The model under review builds one solid part; all positions refer to its coordinate system, in mm. Coordinates: 2 decimals unless noted, no trailing zeros. Write each loop counter-clockwise with the first axis right and the second up, starting at its lowest first coordinate (ties: lowest second). Pieces come first, ordered by that corner, then holes. Notation, with made-up numbers: (70.5, -26.5) - (129.5, -26.5) arc R21 cw to (129.5, -18.5) - close; hole circle Ø9 at (51, 80). An arc over 180 degrees is marked (long way). Put each result on its own line as item: value.
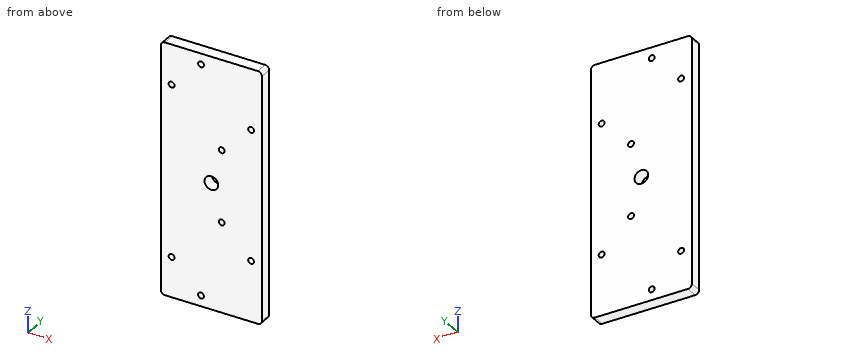
Autodesk Inventor part; units mm, degrees
ref_plane "YZ Plane" through (0, 0, 0) normal (1, 0, 0) x (0, 1, 0)
ref_plane "XZ Plane" through (0, 0, 0) normal (0, 1, 0) x (-1, 0, 0)
ref_plane "XY Plane" through (0, 0, 0) normal (0, 0, 1) x (1, 0, 0)
sketch "Sketch1" plane through (0, 0, 0) normal (0, 1, 0) x (-1, 0, 0)
  line L0 (-25, 62.5) -> (25, 62.5)
  line L1 (25, 62.5) -> (25, -62.5)
  line L2 (25, -62.5) -> (-25, -62.5)
  line L3 (-25, -62.5) -> (-25, 62.5)
  line L4 (-25, 62.5) -> (25, -62.5) construction
  line L5 (25, 62.5) -> (-25, -62.5) construction
  point P0 (0, 0)
  dimension "d0" = 125
  dimension "d1" = 50
extrude "Extrusion1" add sketch "Sketch1" along normal blind 6
sketch "Sketch3" plane through (0, 6, 0) normal (0, 1, 0) x (1, 0, 0)
  line L0 (25, 62.5) -> (-25, 62.5)
  line L1 (-25, -62.5) -> (25, -62.5)
  line L2 (-19.6668, -42.6187) -> (-5.1187, -57.1668)
  line L3 (-5.1187, -57.1668) -> (19.6668, -32.3813)
  line L4 (19.6668, -32.3813) -> (5.1187, -17.8332)
  line L5 (5.1187, -17.8332) -> (-19.6668, -42.6187)
  line L6 (25, -62.5) -> (25, 62.5)
  line L7 (-25, 62.5) -> (-25, -62.5)
  line L8 (5.1187, 17.8332) -> (19.6668, 32.3813)
  line L9 (19.6668, 32.3813) -> (-5.1187, 57.1668)
  line L10 (-5.1187, 57.1668) -> (-19.6668, 42.6187)
  line L11 (-19.6668, 42.6187) -> (5.1187, 17.8332)
  circle A0 centre (-19.6668, -42.6187) radius 1.45
  circle A1 centre (5.1187, -17.8332) radius 1.45
  circle A2 centre (19.6668, -32.3813) radius 1.45
  circle A3 centre (-5.1187, -57.1668) radius 1.45
  circle A4 centre (-19.6668, 42.6187) radius 1.45
  circle A5 centre (-5.1187, 57.1668) radius 1.45
  circle A6 centre (19.6668, 32.3813) radius 1.45
  circle A7 centre (5.1187, 17.8332) radius 1.45
  point P0 (0, 0)
  point P1 (0, -37.5)
  point P2 (0, 37.5)
  point P3 (0, -62.5)
  point P4 (0, 62.5)
  dimension "d5" = 125
  dimension "d7" = 35.052
  dimension "d8" = 20.574
  dimension "d9" = 50
  dimension "d10" = 10.287
  dimension "d11" = 17.526
  dimension "d12" = 35.052
  dimension "d13" = 20.574
  dimension "d14" = 17.526
  dimension "d15" = 10.287
  dimension "d16" = 2.9
  dimension "d17" = 2.9
  dimension "d18" = 2.9
  dimension "d19" = 2.9
  dimension "d20" = 2.9
  dimension "d21" = 2.9
  dimension "d22" = 2.9
  dimension "d23" = 2.9
  dimension "d24" = 25
  dimension "d25" = 25
extrude "Extrusion2" cut sketch "Sketch3" against normal through all contours L5 A0 L2 | L2 A0 L5 | A3 L3 L2 | L2 L3 A3 | A1 L4 L5 | L5 L4 A1 | A2 L4 L3 | L3 L4 A2 | L11 A7 L8 | L8 A7 L11 | A6 L9 L8 | L8 L9 A6 | A4 L10 L11 | L11 L10 A4 | A5 L10 L9 | L9 L10 A5
hole "Hole1" at (0, 6, 0) direction (0, -1, 0) diameter 6.756 end through all
fillet "Fillet1" radius 2 4 edges at (25, 3, 62.5) (25, 3, -62.5) (-25, 3, -62.5) (-25, 3, 62.5)
properties part number "ShuttleValveShelf"
1. To check wall thickness, follow probe 1 along Z at (x, y) = (19.5, 3.8); probe 2 along X at (y, z) = (5.75, 18); probe 3 along Z at (x, y) = (20.5, 3.7). State the ranges of each line that lie inside material, in increasing order.
Determined:
probe 1: z = -62.5 to -33.82, -30.94 to 30.94, 33.82 to 62.5
probe 2: x = -25 to 3.68, 6.56 to 25
probe 3: z = -62.5 to -33.57, -31.19 to 31.19, 33.57 to 62.5
2. Consider section A-A on z = 0. State the section outline as (x, y) points, plus the area to 3 significant figures.
Determined:
outline: (-25, 0) - (-3.38, 0) - (-3.38, 6) - (-25, 6) - close; (3.38, 0) - (25, 0) - (25, 6) - (3.38, 6) - close
area: 259 mm^2
3. Consider section B-B on x = 0. State the section outline as (y, z) points.
Determined:
outline: (0, -62.5) - (6, -62.5) - (6, -3.38) - (0, -3.38) - close; (0, 3.38) - (6, 3.38) - (6, 62.5) - (0, 62.5) - close
4. For pin 1 Ø4.5 at (x, z) = (5.12, 17.83) entering from +Y, flat-tipped, find the tip position at first contact; note if it passes through.
Determined:
pin 1: stops at y = 6
